```python
from build123d import *

# Parameters (mm, degrees)
SZKIC1_W                    = 230
SZKIC1_H                    = 150
DODANIE_WYCI_GNI_CIE1_DEPTH = 5
DODANIE_WYCI_GNI_CIE2_DEPTH = 242
WYTNIJ_WYCI_GNI_CIE1_REACH  = 347.737
SZKIC4_W                    = 30
SZKIC4_H                    = 6
WYTNIJ_WYCI_GNI_CIE2_DEPTH  = 5
SZKIC7_W                    = 2.5
SZKIC7_H                    = 2
WYTNIJ_WYCI_GNI_CIE3_DEPTH  = 145


with BuildPart() as part:
    # Szkic1 → Dodanie-wyciągnięcie1 (new body)
    with BuildSketch(Plane.XY):
        Rectangle(SZKIC1_W, SZKIC1_H)
    extrude(amount=DODANIE_WYCI_GNI_CIE1_DEPTH)

    # Szkic3 → Dodanie-wyciągnięcie2 (add)
    with BuildSketch(Plane.XY.offset(5)):
        Polygon((115, -75), (115, 75), (110, 75), (110, 70), (110, -70), (-110, -70), (-110, 70), (-110, 75), (-115, 75), (-115, -75), align=None)
    extrude(amount=DODANIE_WYCI_GNI_CIE2_DEPTH)

    # Szkic4 → Wytnij-wyciągnięcie1 (cut, up to next)
    with BuildSketch(Plane(origin=(115, 0, 0), x_dir=(0, 0, -1), z_dir=(1, 0, 0)), mode=Mode.PRIVATE) as wytnij_wyci_gni_cie1_sk1:
        with Locations((-223, 72)):
            Rectangle(SZKIC4_W, SZKIC4_H)
    wytnij_wyci_gni_cie1_tool1 = extrude(wytnij_wyci_gni_cie1_sk1.sketch, amount=-WYTNIJ_WYCI_GNI_CIE1_REACH, mode=Mode.PRIVATE) & part.part
    # Szkic4 → Wytnij-wyciągnięcie1 (cut, up to next)
    with BuildSketch(Plane(origin=(115, 0, 0), x_dir=(0, 0, -1), z_dir=(1, 0, 0)), mode=Mode.PRIVATE) as wytnij_wyci_gni_cie1_sk2:
        with Locations((-148, 72)):
            Rectangle(SZKIC4_W, SZKIC4_H)
    wytnij_wyci_gni_cie1_tool2 = extrude(wytnij_wyci_gni_cie1_sk2.sketch, amount=-WYTNIJ_WYCI_GNI_CIE1_REACH, mode=Mode.PRIVATE) & part.part
    # Szkic4 → Wytnij-wyciągnięcie1 (cut, up to next)
    with BuildSketch(Plane(origin=(115, 0, 0), x_dir=(0, 0, -1), z_dir=(1, 0, 0)), mode=Mode.PRIVATE) as wytnij_wyci_gni_cie1_sk3:
        with Locations((-73, 72)):
            Rectangle(SZKIC4_W, SZKIC4_H)
    wytnij_wyci_gni_cie1_tool3 = extrude(wytnij_wyci_gni_cie1_sk3.sketch, amount=-WYTNIJ_WYCI_GNI_CIE1_REACH, mode=Mode.PRIVATE) & part.part
    add(wytnij_wyci_gni_cie1_tool1.solids().sort_by_distance((115, 72, 223))[0], mode=Mode.SUBTRACT)
    add(wytnij_wyci_gni_cie1_tool2.solids().sort_by_distance((115, 72, 148))[0], mode=Mode.SUBTRACT)
    add(wytnij_wyci_gni_cie1_tool3.solids().sort_by_distance((115, 72, 73))[0], mode=Mode.SUBTRACT)

    # Szkic6 → Wytnij-wyciągnięcie2 (cut)
    with BuildSketch(Plane(origin=(115, 0, 0), x_dir=(0, 0, -1), z_dir=(1, 0, 0))):
        Polygon((-11.5, 45), (-11.5, 45.054636006), (-8.5, 45.054636006), (-8.5, 75), (-58, 75), (-58, 69), (-62.5, 69), (-62.5, 45.054636006), (-59.5, 45.054636006), (-59.5, 45), (-55.5, 41), (-55.5, 11), (-15.5, 11), (-15.5, 41), align=None)
        Polygon((-83.5, 45.054636006), (-83.5, 69), (-88, 69), (-88, 75), (-133, 75), (-133, 69), (-137.5, 69), (-137.5, 45.054636006), (-134.5, 45.054636006), (-134.5, 45), (-130.5, 41), (-130.5, 11), (-90.5, 11), (-90.5, 41), (-86.5, 45), (-86.5, 45.054636006), align=None)
        Polygon((-158.5, 45.054636006), (-158.5, 69), (-163, 69), (-163, 75), (-208, 75), (-208, 69), (-212.5, 69), (-212.5, 45.054636006), (-209.5, 45.054636006), (-209.5, 45), (-205.5, 41), (-205.5, 11), (-165.5, 11), (-165.5, 41), (-161.5, 45), (-161.5, 45.054636006), align=None)
    extrude(amount=-WYTNIJ_WYCI_GNI_CIE2_DEPTH, mode=Mode.SUBTRACT)

    # Szkic7 → Wytnij-wyciągnięcie3 (cut)
    with BuildSketch(Plane(origin=(0, 75, 0), x_dir=(1, 0, 0), z_dir=(0, 1, 0))):
        with Locations((-111.25, -244)):
            Rectangle(SZKIC7_W, SZKIC7_H)
        with Locations((111.25, -244)):
            Rectangle(SZKIC7_W, SZKIC7_H)
        Polygon((111, -203), (111, -205.5), (113, -205.5), (113, -203), (115, -203), (115, -168), (113, -168), (113, -165.5), (111, -165.5), (111, -168), (110, -168), (110, -203), align=None)
        Polygon((111, -128), (111, -130.5), (113, -130.5), (113, -128), (115, -128), (115, -93), (113, -93), (113, -90.5), (111, -90.5), (111, -93), (110, -93), (110, -128), align=None)
        Polygon((111, -53), (111, -55.5), (113, -55.5), (113, -53), (115, -53), (115, -18), (113, -18), (113, -15.5), (111, -15.5), (111, -18), (110, -18), (110, -53), align=None)
    extrude(amount=-WYTNIJ_WYCI_GNI_CIE3_DEPTH, mode=Mode.SUBTRACT)


solid = part.part
```
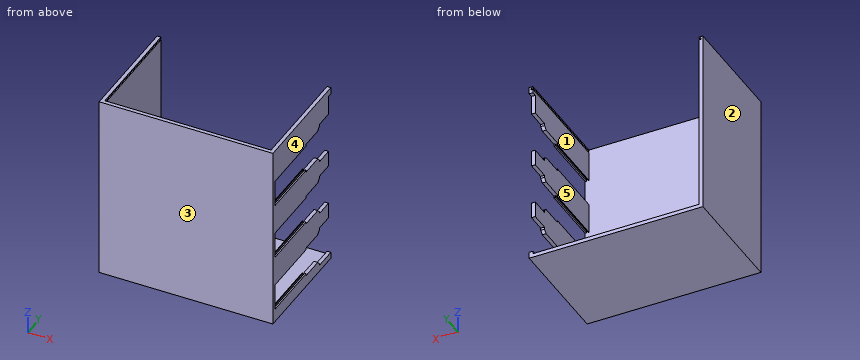
Geometry check sheet. Reference: the model listing, model coordinates, mm. Face numbers are marked on the shaded views. A direction names the side the tool comes from. Coordinates: 2 decimals unless noted, no trailing zeros. Write each loop counter-clockwise with the first axis right and the second up, starting at its lowest first coordinate (ties: lowest second). Pieces come first, ordered by that corner, then holes. Notation, with made-up numbers: M 62.5,-24.75 L 72.5,-24.75 A31 ccw 72.5,13.25 Z; hole C 74.25,30.5 d6. An arc over 180 degrees is marked long. One line per item, written item: value. Start each with the question number.
(1) Scan lines: line 1 along X through (y, z) = (23, 224.5); line 2 along X through (y, z) = (-69, 197); line 3 along Y through (x, z) = (13, 17.5). Record each from-to range of solid material in increasing order. Write a range as [from, to].
(2) Sectioned sample at A-A, the plane y = 32. Enter the section's corners in (x, z), and give its area (3 significant figures).
(3) Sectioned sample at C-C, the plane x = -76. Enter the section's corners in (y, z).
(4) Release check for a two-part mould opening along X. For the marked faces 1, 2 and 3 record: released by +X, released by -X, zero draft, split by the parting line, or undercut.
(5) Sectioned sample at D-D, the plane y = 55. Enter the section's corners in (x, z).
(6) Tool access check on the marked faces 4 and 5. Record the directions out of +Z, -Z, +X, -X, +Y, -Y that give a thin tool (end or side, any length) a straight path to the whole face; none if there is none.
(7) Sectioned sample at B-B, the plane z = 194. Enter the section's corners in (x, y).
(8) Depth check by flat-ended pin: pin 1 (1.5 mm diameter, centred on x = 111.5, y = 59, fed in from -Z); pin 2 (1.6 mm diameter, centred on x = 114, z = 17.5, fed in from +Y); pin 3 (3 mm diameter, centred on y = -45, z = 28.5, fed in from +X); pin 4 (6 mm diameter, centred on x = 32.5, z = 176, fed in from +Y). Enter the tip coordinate at first touch or a pass-through.
Filled sheet:
1. line 1: [-115, -110], [110, 115]
1. line 2: [-115, -110]
1. line 3: [-75, -70]
2. outline: M -115,0 L 115,0 L 115,15.5 L 110,15.5 L 110,5 L -110,5 L -110,243 L -112.5,243 L -112.5,245 L -110,245 L -110,247 L -115,247 Z; M 110,55.5 L 115,55.5 L 115,90.5 L 110,90.5 Z; M 110,130.5 L 115,130.5 L 115,165.5 L 110,165.5 Z; M 110,205.5 L 115,205.5 L 115,247 L 110,247 L 110,245 L 112.5,245 L 112.5,243 L 110,243 Z
2. area: 2,960 mm²
3. outline: M -75,0 L 75,0 L 75,5 L -70,5 L -70,247 L -75,247 Z
4. face 1: undercut
4. face 2: released by -X
4. face 3: zero draft
5. outline: M -115,0 L 115,0 L 115,8.5 L 110,8.5 L 110,5 L -110,5 L -110,243 L -112.5,243 L -112.5,245 L -110,245 L -110,247 L -115,247 Z; M 110,62.5 L 115,62.5 L 115,83.5 L 110,83.5 Z; M 110,137.5 L 115,137.5 L 115,158.5 L 110,158.5 Z; M 110,212.5 L 115,212.5 L 115,247 L 110,247 L 110,245 L 112.5,245 L 112.5,243 L 110,243 Z
6. face 4: +Z, -Z, +X, +Y, -Y
6. face 5: +Z, +Y
7. outline: M -115,-75 L 115,-75 L 115,-70 L -110,-70 L -110,75 L -115,75 Z
8. pin 1: z = 0
8. pin 2: y = 11
8. pin 3: x = -110
8. pin 4: y = -70
